Study the drawing (mm; zero at the part's minimum x, y, z) and answer. Coordinates: 2 decimals unless noted, no trailing zeros. Loops run counter-clockwise (first coordinate to the right, second up) from the corner with the lowest first, then second, coordinate; pieces in that order, holes last. Notation, with made-up numbers: (47, 7.5) - (70, 7.5) arc R24 ccw to (70, 25.5) - close; hole circle Ø8 at (61, 85). An arc over 180 degrees is marked (long way). Write each question's results on one line, items separated by ' | '. Start each with the question number.
(1) Given pin 1 Ø1.5 at (x, z) = (7, 6.5) entering from -Y; pin 2 Ø6 at (x, z) = (1.5, 5.5) entering from +Y; pin 3 Ø6 at (x, y) = (7, 4) entering from -Z; pin 4 Ø1 at (y, z) = (1.5, 4) entering from -X, each flat-ended and moving along its own axis, determine where each tip first touches the part or whether it passes through.
(2) Consider line 1 (Y direction, x = 6, z = 3.5); line 2 (X direction, y = 7.5, z = 9); line 3 (X direction, y = 6.75, z = 5.25). Determine where each line is inside the solid, lowest interval first. Write a range as from..to.
(3) Determine the mould class of the marked faces 1, 2 and 3 for opening direction Y: released by +Y, released by -Y, zero draft, split by the parting line, or undercut.
(4) Find section A-A on x = 6. Determine the outline of the cut face in (y, z), then the cut area to 3 significant figures.
(5) Find section C-C on z = 12. Determine the outline of the cut face in (x, y).
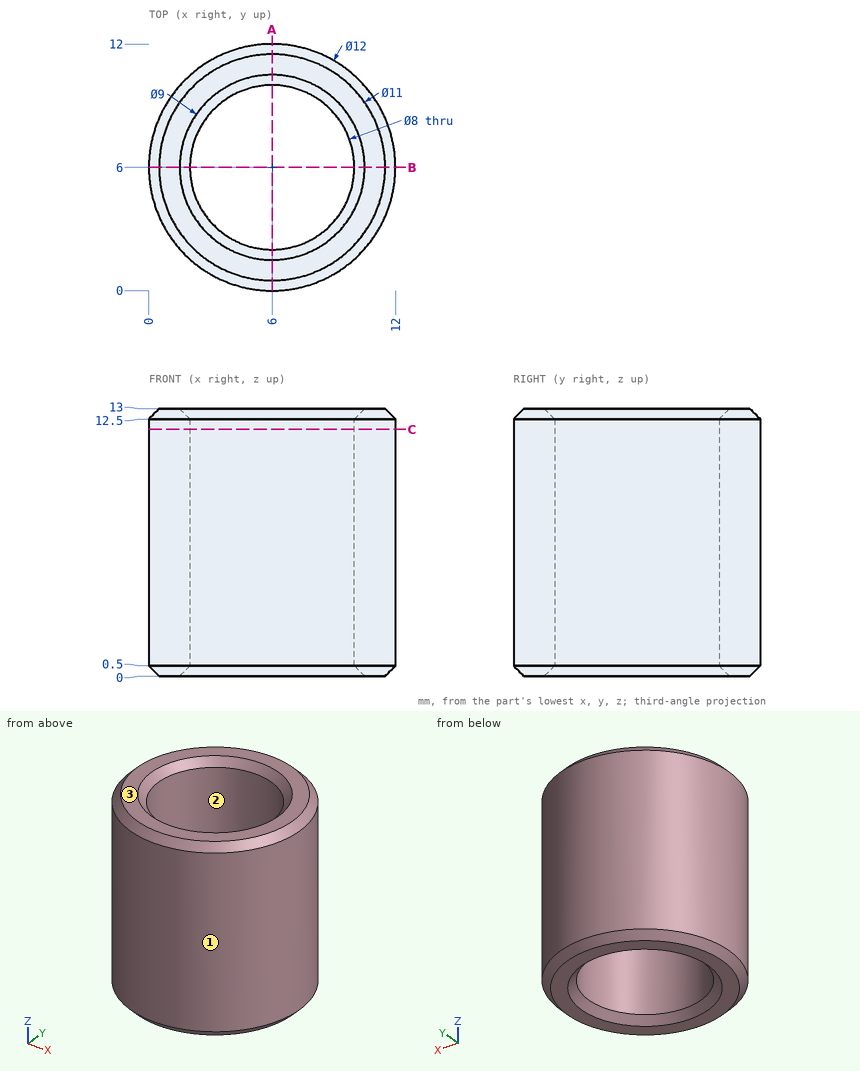
Values:
1) pin 1: stops at y = 0.01 | pin 2: stops at y = 11.81 | pin 3: stops at z = 0 | pin 4: stops at x = 1.53
2) line 1: y = 0..2, 10..12 | line 2: x = 0.19..2.29, 9.71..11.81 | line 3: x = 0.05..2.07, 9.93..11.95
3) face 1: split by the parting line | face 2: undercut | face 3: zero draft
4) outline: (0, 0.5) - (0.5, 0) - (1.5, 0) - (2, 0.5) - (2, 12.5) - (1.5, 13) - (0.5, 13) - (0, 12.5) - close; (10, 0.5) - (10.5, 0) - (11.5, 0) - (12, 0.5) - (12, 12.5) - (11.5, 13) - (10.5, 13) - (10, 12.5) - close | area: 51.0 mm²
5) outline: circle Ø12 at (6, 6); hole circle Ø8 at (6, 6)
